Geometry: see drawing. Coordinates: mm, zero at the bounding-box minimum. A direction names the side the tool comes from. Coordinates: 2 decimals unless noted, no trailing zeros. Loops run counter-clockwise (first coordinate to the right, second up) from the corner with the lowest first, then second, coordinate; pieces in that order, holes last. Notation, with made-up numbers: M 9.25,27 L 14.25,27 A14 ccw 14.25,36 Z; hole C 74.25,-31.5 d9. An arc over 180 degrees is marked long. One line per question, with ' | ' between items. Start each with the question number.
1. Section query D-D, the plane x = 56. Output: boundary loops of the cut face in (y, z).
2. Pin query (flat end, axial travel): P1, Ø4, axis at x = 47, y = 4, coming from the -Z side (3 decimals); P2, Ø4, axis at y = 5.5, z = 53.5, coming from the -X side; P3, Ø5, axis at y = 6, z = 34.5, coming from the -X side. Return the tip coordinate at first contact, or that it passes through.
3. Section query B-B, the plane z = 59. Output: boundary loops of the cut face in (x, y) (1 decimal).
4. Section query C-C, the plane z = 42. State how many separate pieces and enclosed holes the cut face has.
5. Mould query, pull axis Z, two halves, no side actions, for the marked faces 6, 7, 8 and 9. Classes: pulls with the +Z half, pulls with the -Z half, needs draft (parallel to the pull), parting line crosses it, or undercut.
6. Ray query, probe 1 along X at (y, z) = (6, 61) (1 decimal); probe 2 along X at (y, z) = (11, 22) (1 decimal); probe 3 along X at (y, z) = (9, 27) (1 decimal). Return the intervals inside material, ascending.
7. Access query for the marked faces 1, 2, 3, 4 and 5. Directions: +Z, -Z, +X, -X, +Y, -Y. A direction counts if a zero-diameter tool reaches every point of the face in a straight line with its end or side. Return the directions, or none.
8. Section query A-A, the plane x = 6.35. Output: boundary loops of the cut face in (y, z) (1 decimal).
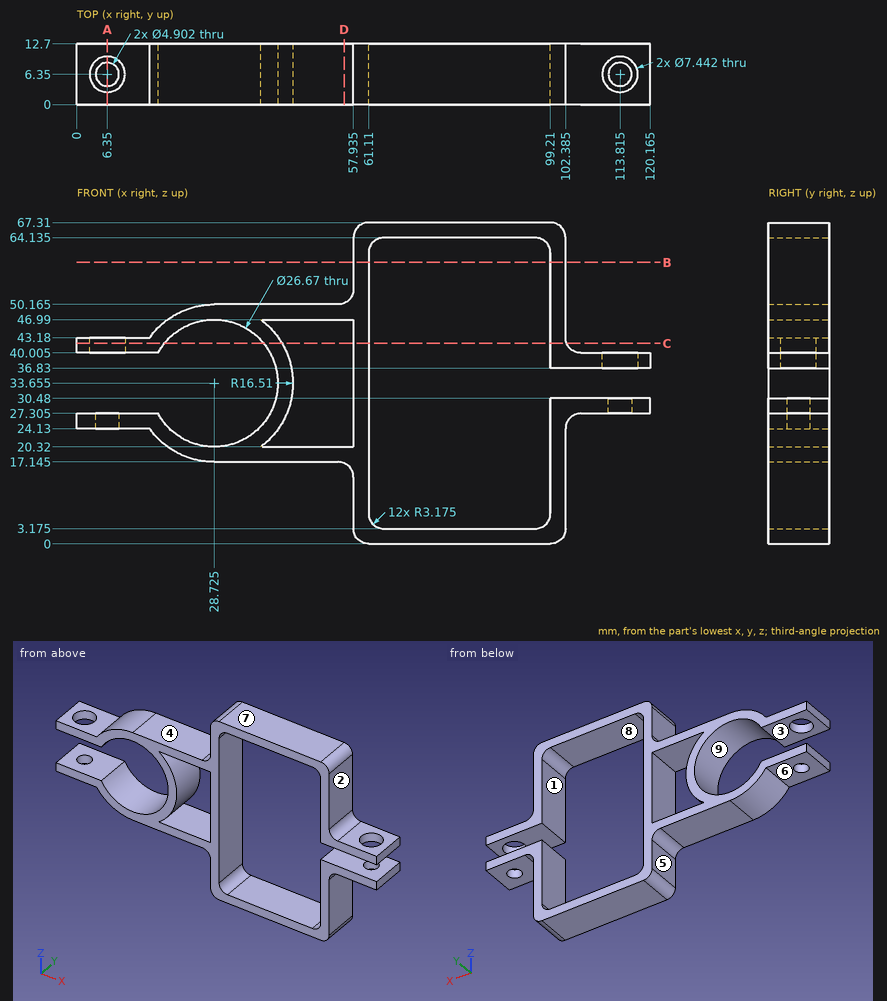
Taken from the geometry:
1) outline: M 0,16.89 L 12.7,16.89 L 12.7,20.32 L 0,20.32 Z; M 0,46.99 L 12.7,46.99 L 12.7,50.42 L 0,50.42 Z
2) P1: z = 17.145 | P2: x = 57.35 | P3: x = 41.63
3) outline: M 57.9,0 L 61.1,0 L 61.1,12.7 L 57.9,12.7 Z; M 99.2,0 L 102.4,0 L 102.4,12.7 L 99.2,12.7 Z
4) separate pieces: 4 | enclosed holes: 1
5) face 6: pulls with the -Z half | face 7: pulls with the +Z half | face 8: undercut | face 9: undercut
6) probe 1: 57.9 to 61.1, 99.2 to 102.4 | probe 2: 17 to 22.2, 35.2 to 40.4, 57.9 to 61.1, 99.2 to 102.4 | probe 3: 0 to 17.2, 40.3 to 43.8, 57.9 to 61.1, 99.2 to 104.2
7) face 1: +Y, -Y | face 2: +Z, +X, +Y, -Y | face 3: -X, +Y, -Y | face 4: +Z, -X, +Y, -Y | face 5: -Z, -X, +Y, -Y
8) outline: M 0,24.1 L 3.9,24.1 L 3.9,27.3 L 0,27.3 Z; M 0,40 L 2.6,40 L 2.6,43.2 L 0,43.2 Z; M 8.8,24.1 L 12.7,24.1 L 12.7,27.3 L 8.8,27.3 Z; M 10.1,40 L 12.7,40 L 12.7,43.2 L 10.1,43.2 Z
